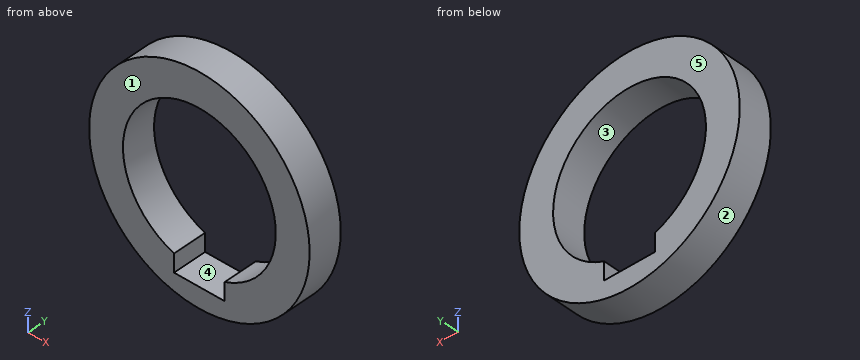
from build123d import *

# Parameters (mm, degrees)
SKETCH1_R      = 32.6
EXTRUDE1_DEPTH = 10


with BuildPart() as part:
    # Sketch1 → Extrude1 (new body)
    with BuildSketch(Plane(origin=(0, 0, 0), x_dir=(1, 0, 0), z_dir=(0, 1, 0))):
        Circle(SKETCH1_R)
        with BuildLine():
            Line((-7.5, 26.6), (-7.5, 21.319240137))
            ThreePointArc((-7.5, 21.319240137), (0, -22.6), (7.5, 21.319240137))
            Line((7.5, 21.319240137), (7.5, 26.6))
            Line((7.5, 26.6), (-7.5, 26.6))
        make_face(mode=Mode.SUBTRACT)
    extrude(amount=EXTRUDE1_DEPTH)


solid = part.part
Build history of the part. All positions in model axes, mm. Face numbers are marked on the shaded views. A direction names the side the tool comes from. Give positions to 0.01 mm unless a question says otherwise; leave off trailing zeros. Order: outer loops, then holes, each group sorted by start corner. A loop starts at its lowest first (then second) coordinate and runs counter-clockwise, first axis right, second up. Notation, with made-up numbers: M -40,-9.5 L -20,-9.5 A22 cw -20,27.5 Z; hole C -23.5,6 d2. An arc over 180 degrees is marked long. Put each result on its own line as item: value.
Item 1: Flat gauge pins, fed straight in: pin 1 Ø4 at (y, z) = (5, -24.5) entering from -X; pin 2 Ø5 at (x, y) = (17.5, 8.5) entering from -Z; pin 3 Ø5 at (y, z) = (8.5, -24.5) entering from +X. Where does each tip first touch, or does it go through?
From the geometry:
pin 1: stops at x = -23.59
pin 2: stops at z = -28.94
pin 3: stops at x = 24.06
Item 2: Slice it at D-D, the plane z = 27.5. Write the cut outline in (x, y), plus the area to 3 significant figures.
From the geometry:
outline: M -17.51,0 L 17.51,0 L 17.51,10 L -17.51,10 Z
area: 350 mm2
Item 3: 3-axis set-ups, long thin cutter, end or side, ignore diameter. For the marked faces 4 and 5: which of +Z, -Z, +X, -X, +Y, -Y reach the whole face in a straight line?
From the geometry:
face 4: +Y, -Y
face 5: +Z, -Z, +X, -X, +Y
Item 4: Slice it at C-C, the plane y = 6.25. Write the cut outline in (x, z), plus the area to 3 significant figures.
From the geometry:
outline: C 0,0 d65.2; hole M -7.5,-26.6 L 7.5,-26.6 L 7.5,-21.32 A22.6 ccw long -7.5,-21.32 Z
area: 1,670 mm2
Item 5: Slice it at B-B, the plane z = 4.5. Write the cut outline in (x, y), plus the area to 3 significant figures.
From the geometry:
outline: M -32.29,0 L -22.15,0 L -22.15,10 L -32.29,10 Z; M 22.15,0 L 32.29,0 L 32.29,10 L 22.15,10 Z
area: 203 mm2
Item 6: Slice it at A-A, the plane x = 0. Write the cut outline in (y, z).
From the geometry:
outline: M 0,-32.6 L 10,-32.6 L 10,-26.6 L 0,-26.6 Z; M 0,22.6 L 10,22.6 L 10,32.6 L 0,32.6 Z
Item 7: Two-plate mould, pull along Z, no slides. Class the marked faces 1, 2 and 3: +Z half, -Z half, draft (parallel to the pull), parting line (faces both ways), or undercut.
From the geometry:
face 1: draft
face 2: parting line
face 3: undercut
Item 8: Probe line 1 (X direction, y = 6, z = 0); line 2 (Z direction, x = 0, y = 3.75); line 3 (X direction, y = 0.75, z = -23.5). List the from-to ranges inside material, lowest first. Write a range as [from, to].
From the geometry:
line 1: x = [-32.6, -22.6], [22.6, 32.6]
line 2: z = [-32.6, -26.6], [22.6, 32.6]
line 3: x = [-22.59, -7.5], [7.5, 22.59]
